```python
from build123d import *


with BuildPart() as part:
    # Sketch1 → Revolve1 (revolve)
    with BuildSketch(Plane.XY):
        Polygon((-180, 0), (0, 0), (0, 50), (-60, 50), (-60, 30), (-100, 30), (-100, 10), (-180, 10), align=None)
        Polygon((0, 0), (180, 0), (180, 10), (100, 10), (100, 30), (60, 30), (60, 50), (0, 50), align=None)
    revolve(axis=Axis((180, 0, 0), (-1, 0, 0)))


solid = part.part
```
The listing builds one solid part. Answer for the finished solid, in the listing's coordinates (mm). A direction names the side the tool comes from. Coordinates: 2 decimals unless noted, no trailing zeros. Write each loop counter-clockwise with the first axis right and the second up, starting at its lowest first coordinate (ties: lowest second). Pieces come first, ordered by that corner, then holes.
Q1. Section A-A, the plane y = 0 is taken. Write down the section's boundary in (x, z), then the cut area to 3 significant figures.
Returned:
outline: (-180, -10) - (-100, -10) - (-100, -30) - (-60, -30) - (-60, -50) - (60, -50) - (60, -30) - (100, -30) - (100, -10) - (180, -10) - (180, 10) - (100, 10) - (100, 30) - (60, 30) - (60, 50) - (-60, 50) - (-60, 30) - (-100, 30) - (-100, 10) - (-180, 10) - close
area: 20,000 mm2
Q2. Which of the six approach directions +Z, -Z, +X, -X, +Y, -Y give full straight-line access (tool end or side, diameter ignored) to faces 1 (the flat face through (-60, 22, 22)), 2 (the flat face through (60, -22, 22)), 3 (the flat face through (-180, 0, 0))?
Returned:
face 1: -X
face 2: +X
face 3: +Z, -Z, -X, +Y, -Y
Q3. Section D-D, the plane x = 31.5 is taken. Write down the section's boundary in (y, z), then the cut area to 3 significant figures.
Returned:
outline: circle Ø100 at (0, 0)
area: 7,850 mm2
Q4. Find the intervals of material crossed by line 1 along X through (y, z) = (-12, 42); line 2 along X through (y, z) = (-4.5, 29.5); line 3 along Y through (x, z) = (-16, -40), in increasing order.
Returned:
line 1: x = -60 to 60
line 2: x = -100 to 100
line 3: y = -30 to 30
Q5. Given P1, Ø1, axis at x = 37, z = -36, coming from the +Y side; P2, Ø4, axis at y = 7.5, z = -39.5, coming from the -X side; P3, Ø12, axis at y = -15.5, z = 28.5, coming from the +X side, each flat-ended and moving along its own axis, determine where each tip first touches the part or whether it passes through.
Returned:
P1: stops at y = 35.21
P2: stops at x = -60
P3: stops at x = 100
Q6. Section C-C, the plane x = 77 is taken. Write down the section's boundary in (y, z).
Returned:
outline: circle Ø60 at (0, 0)
